from build123d import *

# Parameters (mm, degrees)
F0_R     = 11
F0_R_2   = 2
F0_R_3   = 2.5
F1_DEPTH = 5


with BuildPart() as f1:
    # F0 (on Front) → F1 (new body)
    with BuildSketch(Plane.XZ):
        with Locations((58, 0)):
            Circle(F0_R)
        with BuildLine():
            ThreePointArc((0, 30.311465), (-30.311465, 0), (0, -30.311465))
            Line((0, -30.311465), (83, -20))
            Line((83, -20), (83, 0))
            Line((83, 0), (83, 20))
            Line((83, 20), (0, 30.311465))
        make_face()
        with Locations((-15.5, -15.5)):
            Circle(F0_R_2, mode=Mode.SUBTRACT)
        with Locations((0, -25)):
            Circle(F0_R_3, mode=Mode.SUBTRACT)
        with Locations((15.5, -15.5)):
            Circle(F0_R_2, mode=Mode.SUBTRACT)
        with Locations((78, -15)):
            Circle(F0_R_3, mode=Mode.SUBTRACT)
        Circle(F0_R, mode=Mode.SUBTRACT)
        with Locations((-15.5, 15.5)):
            Circle(F0_R_2, mode=Mode.SUBTRACT)
        with Locations((15.5, 15.5)):
            Circle(F0_R_2, mode=Mode.SUBTRACT)
        with Locations((0, 25)):
            Circle(F0_R_3, mode=Mode.SUBTRACT)
        with Locations((58, 0)):
            Circle(F0_R, mode=Mode.SUBTRACT)
        with Locations((78, 15)):
            Circle(F0_R_3, mode=Mode.SUBTRACT)
    extrude(amount=F1_DEPTH)


solid = f1.part
The model under review builds one solid part; all positions refer to its coordinate system, in mm. Round coordinates to 2 decimals unless told otherwise and drop trailing zeros. Order: outer loops, then holes, each group sorted by start corner. A loop starts at its lowest first (then second) coordinate and runs counter-clockwise, first axis right, second up. Notation, with made-up numbers: (-35, 21) -> (7, 21) arc R19 ccw to (7, 32) -> close; hole circle Ø4 at (51, 20). An arc over 180 degrees is marked (long way). Return JSON: item names as keys, results as strings.
1. The part is to be moulded in two halves that separate along X. For faces 1 (the face through (-30.304, -2.465, 0.667)), 2 (the face through (26, -5, 0)), 3 (the face through (15.24, -2.465, -13.517)), 4 (the face through (40.919, -2.465, -25.228)), say which applies: +X half, -X half, draft (parallel to the pull), parting line (faces both ways), or undercut.
Answer block:
{"face 1": "-X half", "face 2": "draft", "face 3": "undercut", "face 4": "+X half"}
2. Insertion check: P1, Ø1, axis at x = -14.5, y = -1.5, coming from the +Z side; P2, Ø1, axis at x = 50.5, y = -1, coming from the -Z side; P3, Ø1, axis at x = -7.5, y = -4, coming from the +Z side. Each pin has a flat end and moves straight along its axis. Give the tip position at first contact, or say it passes through.
Answer block:
{"P1": "stops at z = 26.88", "P2": "stops at z = -24.1", "P3": "stops at z = 29.49"}
3. Take a section at B-B (x = 50). Write out the cut boundary in (y, z).
Answer block:
{"outline": "(-5, -24.1) -> (0, -24.1) -> (0, -7.55) -> (-5, -7.55) -> close; (-5, 7.55) -> (0, 7.55) -> (0, 24.1) -> (-5, 24.1) -> close"}
4. Take a section at C-C (z = -7.5). Write out the cut boundary in (x, y), then the cut area to 3 significant figures.
Answer block:
{"outline": "(-29.37, -5) -> (-8.05, -5) -> (-8.05, 0) -> (-29.37, 0) -> close; (8.05, -5) -> (49.95, -5) -> (49.95, 0) -> (8.05, 0) -> close; (66.05, -5) -> (83, -5) -> (83, 0) -> (66.05, 0) -> close", "area": "401 mm²"}
5. For L1, parallel to X at y = -0.4, z = -0.5; L2, parallel to X at y = -3.45, z = -6; L3, parallel to Z at x = 15.5, y = -3.2, list the stretches that pass through material, from the lowest coordinate up. Write a range as [from, to].
Answer block:
{"L1": "x = [-30.31, -10.99], [10.99, 47.01], [68.99, 83]", "L2": "x = [-29.71, -9.22], [9.22, 48.78], [67.22, 83]", "L3": "z = [-28.39, -17.5], [-13.5, 13.5], [17.5, 28.39]"}
6. Take a section at A-A (y = -1.75). State how many separate pieces and enclosed holes the cut face has, then the cut area to 3 significant figures.
Answer block:
{"separate pieces": "1", "enclosed holes": "10", "area": "4,730 mm²"}
7. Take a section at D-D (z = -25). Write out the cut boundary in (x, y).
Answer block:
{"outline": "(-17.14, -5) -> (-2.5, -5) -> (-2.5, 0) -> (-17.14, 0) -> close; (2.5, -5) -> (42.75, -5) -> (42.75, 0) -> (2.5, 0) -> close"}
